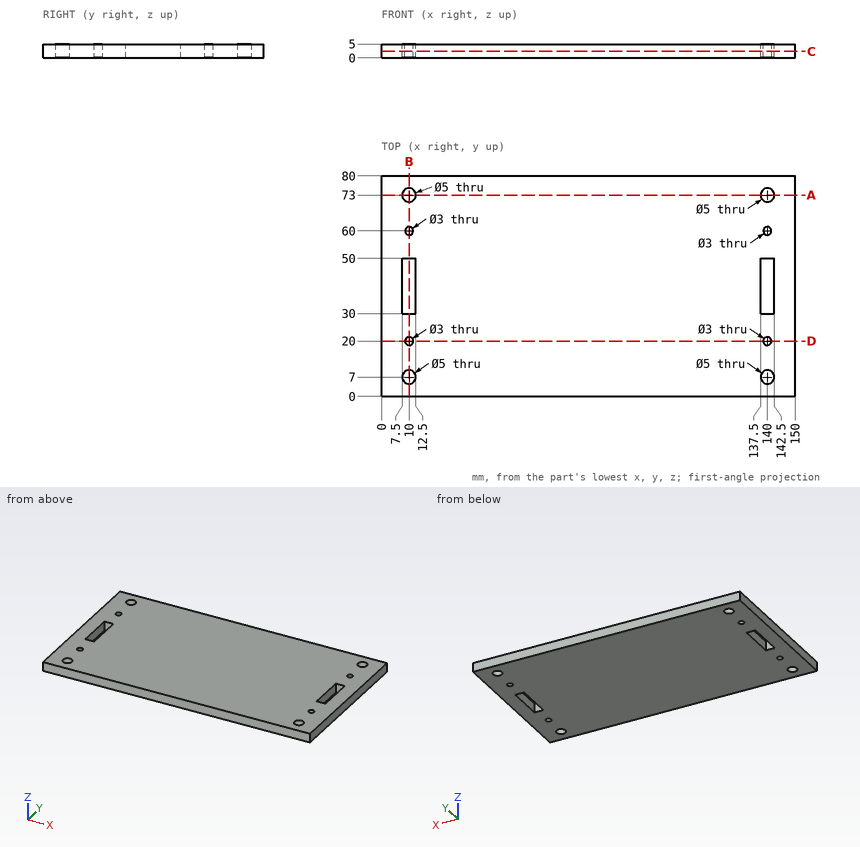
Verification items for this drawing (mm, ordinates from the low corner). Coordinates: 2 decimals unless noted, no trailing zeros. Loops run counter-clockwise (first coordinate to the right, second up) from the corner with the lowest first, then second, coordinate; pieces in that order, holes last. Notation, with made-up numbers: (-18, 18.5) - (20, 18.5) arc R16 cw to (20, 41.5) - close; hole circle Ø8 at (34.5, 55). An arc over 180 degrees is marked (long way). Answer as a JSON object with one key per item and string values.
(1) Scan line: line 1 along Y through (x, z) = (140, 3.05). Record every from-to range of solid material in increasing order.
Response:
{"line 1": "y = 0 to 4.5, 9.5 to 18.5, 21.5 to 30, 50 to 58.5, 61.5 to 70.5, 75.5 to 80"}
(2) Cross-section at C-C, the plane z = 2.3. Count the separate pieces of the cut face and the enclosed holes in it, then the cut area to 3 significant figures.
Response:
{"separate pieces": "1", "enclosed holes": "10", "area": "11,700 mm²"}
(3) Cross-section at B-B, the plane x = 10. Record the boundary of the cut face in (y, z).
Response:
{"outline": "(0, 0) - (4.5, 0) - (4.5, 5) - (0, 5) - close; (9.5, 0) - (18.5, 0) - (18.5, 5) - (9.5, 5) - close; (21.5, 0) - (30, 0) - (30, 5) - (21.5, 5) - close; (50, 0) - (58.5, 0) - (58.5, 5) - (50, 5) - close; (61.5, 0) - (70.5, 0) - (70.5, 5) - (61.5, 5) - close; (75.5, 0) - (80, 0) - (80, 5) - (75.5, 5) - close"}
(4) Cross-section at D-D, the plane y = 20. Record the boundary of the cut face in (x, z), then the cut area to 3 significant figures.
Response:
{"outline": "(0, 0) - (8.5, 0) - (8.5, 5) - (0, 5) - close; (11.5, 0) - (138.5, 0) - (138.5, 5) - (11.5, 5) - close; (141.5, 0) - (150, 0) - (150, 5) - (141.5, 5) - close", "area": "720 mm²"}
(5) Cross-section at A-A, the plane y = 73. Record the boundary of the cut face in (x, z).
Response:
{"outline": "(0, 0) - (7.5, 0) - (7.5, 5) - (0, 5) - close; (12.5, 0) - (137.5, 0) - (137.5, 5) - (12.5, 5) - close; (142.5, 0) - (150, 0) - (150, 5) - (142.5, 5) - close"}
